```python
from build123d import *

# Parameters (mm, degrees)
F0_W     = 70
F0_H     = 20
F1_DEPTH = 10
F2_R     = 5
F3_R     = 1.8
F4_DEPTH = 20
F5_R     = 1.8
F6_DEPTH = 20


with BuildPart() as f1:
    # F0 (on Top) → F1 (new body)
    with BuildSketch(Plane.XY):
        with Locations((-45.893969, 6.072203)):
            Rectangle(F0_W, F0_H)
        Polygon((-10.893969, 16.072203), (-10.893969, -3.927797), (32.407302, 21.072203), (23.747048, 36.072203), align=None)
        Polygon((23.747048, 36.072203), (32.407302, 21.072203), (37.188711, 52.469358), (26.193698, 52.138151), align=None)
        Polygon((26.193698, 52.138151), (37.188711, 52.469358), (31.691205, 63.501806), (22.561267, 58.952328), align=None)
    extrude(amount=F1_DEPTH)

    # F2
    f2_edges = [f1.edges().sort_by_distance(p)[0] for p in [
        (-80.893969, 16.072203, 5),
        (-80.893969, -3.927797, 5),
    ]]
    fillet(f2_edges, radius=F2_R)

    # F3 (on face) → F4 (cut)
    with BuildSketch(Plane.XY.offset(10)):
        with Locations((-76.693969, 6.072203)):
            Circle(F3_R)
    extrude(amount=-F4_DEPTH, mode=Mode.SUBTRACT)

    # F5 (on face) → F6 (cut)
    with BuildSketch(Plane.XY.offset(10)):
        with Locations((-10.893969, 6.272203)):
            Circle(F5_R)
    extrude(amount=-F6_DEPTH, mode=Mode.SUBTRACT)


solid = f1.part
```
Geometry check sheet. Reference: the model listing, model coordinates, mm. A direction names the side the tool comes from. Round coordinates to 2 decimals unless told otherwise and drop trailing zeros. Loops run counter-clockwise (first coordinate to the right, second up) from the corner with the lowest first, then second, coordinate; pieces in that order, holes last. Notation, with made-up numbers: (-36.5, 86.5) - (14.5, 86.5) arc R32 ccw to (14.5, 124.5) - close; hole circle Ø11 at (34, 56.5). An arc over 180 degrees is marked (long way). Write item = value, one per line. Start each with the question number.
1. Section check A-A on z = 7.5. Enter the section's corners in (x, y), then the cut area to 3 significant figures.
2. Section check C-C on x = 14. Enter the section's corners in (y, z).
3. Thickness scan on line 1 (Y direction, x = -30.5, z = 1.75); line 2 (X direction, y = 22, z = 5); line 3 (X direction, y = 13, z = 7). Record the ranges inside material, lowest first.
4. Section check B-B on y = 33. Enter the section's corners in (x, z).
5. Mould release check, pull along Y, two halves, no side actions. Record for faces 1 (the face through (-75.031, 5.383, 5.07)), 2 (the face through (24.987, 44.218, 4.93)), 3 (the face through (-79.47, -2.42, 5.07)), 4 (the face through (-80.894, 6, 5)): released by +Y, released by -Y, zero draft, split by the parting line, or undercut.
6. Depth check by flat-ended pin: pin 1 (1.5 mm diameter, centred on y = 23.5, z = 4.5, fed in from +X); pin 2 (1 mm diameter, centred on x = -30, z = 2.5, fed in from +Y); pin 3 (1 mm diameter, centred on y = 10.5, z = 5, fed in from +X). Enter the tip coordinate at first touch or a pass-through.
7. Set-up check for faces 5 (the face through (-44, 16.072, 5)), 6 (the face through (24.352, 55.593, 4.93)), 7 (the face through (-23, 15, 10)): record each of +Z, -Z, +X, -X, +Y, -Y from which the full face is reachable in a straight line by a thin tool's end or side.
Working result:
q1.outline = (-80.89, 1.07) arc R5 ccw to (-75.89, -3.93) - (-10.89, -3.93) - (32.41, 21.07) - (37.19, 52.47) - (31.69, 63.5) - (22.56, 58.95) - (26.19, 52.14) - (23.75, 36.07) - (-10.89, 16.07) - (-75.89, 16.07) arc R5 ccw to (-80.89, 11.07) - close; hole circle Ø3.6 at (-76.69, 6.07); hole circle Ø3.6 at (-10.89, 6.27)
q1.area = 2,510 mm^2
q2.outline = (10.44, 0) - (30.44, 0) - (30.44, 10) - (10.44, 10) - close
q3.line_1 = -3.93 to 16.07
q3.line_2 = -0.63 to 32.55
q3.line_3 = -80.51 to 18.43
q4.outline = (18.43, 0) - (34.22, 0) - (34.22, 10) - (18.43, 10) - close
q5.face_1 = undercut
q5.face_2 = undercut
q5.face_3 = released by -Y
q5.face_4 = zero draft
q6.pin_1 = 32.89
q6.pin_2 = 16.07
q6.pin_3 = 14.96
q7.face_5 = +Z, -Z, -X, +Y
q7.face_6 = +Z, -Z, -X
q7.face_7 = +Z, +X, -X, +Y, -Y
